Check sheet for the modelled part. Datum: model origin and axes. Units: mm. A direction names the side the tool comes from. Coordinates: 2 decimals unless noted, no trailing zeros. Order: outer loops, then holes, each group sorted by start corner. A loop starts at its lowest first (then second) coordinate and runs counter-clockwise, first axis right, second up. Notation, with made-up numbers: M -32,3 L -14,3 A30 ccw -14,25 Z; hole C 56,52 d4. An arc over 180 degrees is marked long. Answer in a Markdown table with one row per item. Add a question column.
Autodesk Inventor part; units mm, degrees
ref_plane "YZ Plane" through (0, 0, 0) normal (1, 0, 0) x (0, 1, 0)
ref_plane "XZ Plane" through (0, 0, 0) normal (0, 1, 0) x (-1, 0, 0)
ref_plane "XY Plane" through (0, 0, 0) normal (0, 0, 1) x (1, 0, 0)
sketch "Эскиз1" plane through (0, 0, 0) normal (0, 1, 0) x (-1, 0, 0)
  line L0 (-7.5, -10) -> (7.5, -10)
  line L1 (7.5, -10) -> (7.5, 4)
  line L2 (1.5, 10) -> (-1.5, 10)
  line L3 (-7.5, 4) -> (-7.5, -10)
  line L4 (-7.5, -10) -> (7.5, 10) construction
  line L5 (7.5, -10) -> (-7.5, 10) construction
  arc A0 (7.5, 4) -> (1.5, 10) centre (1.5, 4) ccw
  arc A1 (-1.5, 10) -> (-7.5, 4) centre (-1.5, 4) ccw
  line L6 (0, -10) -> (5, -10)
  point P0 (0, 0)
  dimension "d0" = 15
  dimension "d1" = 20
  dimension "d2" = 6
  dimension "d3" = 6
extrude "Выдавливание1" add sketch "Эскиз1" along normal blind 9
sketch "Эскиз3" plane through (7.5, 0, -10) normal (0, 0, -1) x (-1, 0, 0)
  line L0 (0, 0) -> (0, 9)
  line L1 (15, 0) -> (9, 0)
  line L2 (0, 9) -> (15, 9)
  line L3 (15, 9) -> (15, 0)
  line L4 (15, 0) -> (0, 0)
  line L5 (0, 0) -> (0, 9)
  circle A0 centre (7.5, 4.5) radius 4.5
  point P0 (7.5, 0)
  dimension "d11" = 9
  dimension "d12" = 4.5
extrude "Выдавливание3" add sketch "Эскиз3" along normal blind 20 contours A0
properties part number "moroshenka"
1. Go/stop test with flat-tipped pins: pin 1 Ø1.5 at (x, y) = (4.5, 6) entering from +Z; pin 2 Ø2 at (x, y) = (3.5, 6) entering from +Z; pin 3 Ø1 at (x, z) = (-2, -22.5) entering from +Y. Record where each tip stops, or that it passes through.
2. Section check C-C on z = -22.5. Enter the section's corners in (x, y).
3. Set-up check for faces 1 (the flat face through (0, 9, 0)), 2 (the cylindrical face through (3.6, 7.2, -19.9)): record each of +Z, -Z, +X, -X, +Y, -Y from which the full face is reachable in a straight line by a thin tool's end or side.
4. Scan lines: line 1 (X direction, y = 4.75, z = -20.5); line 2 (Z direction, x = 7, y = 3.75); line 3 (Z direction, x = -2.75, y = 3.25). Record each from-to range of solid material in increasing order.
5. Section check D-D on x = -3. Enter the section's corners in (y, z), then the cut area to 3 significant figures.
6. Section check B-B on x = 3.75. Enter the section's corners in (y, z), then the cut area to 3 significant figures.
7. Section check A-A on y = 4.5. Enter the section's corners in (x, z).
Result sheet:
| question | item | result |
|---|---|---|
| 1 | pin 1 | z = 9.56 |
| 1 | pin 2 | z = 9.92 |
| 1 | pin 3 | y = 8.74 |
| 2 | outline | C 0,4.5 d9 |
| 3 | face 1 | +Z, -Z, +X, -X, +Y |
| 3 | face 2 | -Z |
| 4 | line 1 | -4.49 to 4.49 |
| 4 | line 2 | -10 to 6.4 |
| 4 | line 3 | -30 to 9.87 |
| 5 | outline | M 0,-10 L 1.15,-10 L 1.15,-30 L 7.85,-30 L 7.85,-10 L 9,-10 L 9,9.81 L 0,9.81 Z |
| 5 | area | 312 mm^2 |
| 6 | outline | M 0,-10 L 2.01,-10 L 2.01,-30 L 6.99,-30 L 6.99,-10 L 9,-10 L 9,9.56 L 0,9.56 Z |
| 6 | area | 276 mm^2 |
| 7 | outline | M -7.5,-10 L -4.5,-10 L -4.5,-30 L 4.5,-30 L 4.5,-10 L 7.5,-10 L 7.5,4 A6 ccw 1.5,10 L -1.5,10 A6 ccw -7.5,4 Z |
